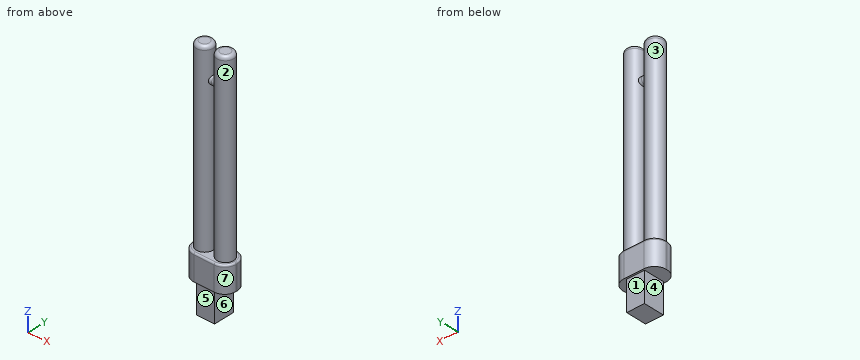
```python
from build123d import *

# Parameters (mm, degrees)
F0_R          = 6.096
F1_DEPTH      = 134.62
F2_R          = 2.921
F3_DEPTH      = 5.08
F3_DEPTH_BACK = 5.08
F4_R          = 2.54
F6_DEPTH      = 19.05
F7_R          = 1.27
F8_W          = 13.208
F8_H          = 15.24
F9_DEPTH      = 21.844


with BuildPart() as f1:
    # F0 (on Top) → F1 (new body)
    with BuildSketch(Plane.XY):
        with Locations((7.62, 0)):
            Circle(F0_R)
        with Locations((-7.62, 0)):
            Circle(F0_R)
    extrude(amount=F1_DEPTH)

    # F2 (on Right) → F3 (join, two sides)
    with BuildSketch(Plane.YZ) as f3_sk:
        with Locations((0, 111.602642)):
            Circle(F2_R)
    extrude(amount=F3_DEPTH)
    extrude(f3_sk.sketch, amount=-F3_DEPTH_BACK)

    # F4
    f4_edges = [f1.edges().sort_by_distance(p)[0] for p in [
        (-13.716, 0, 134.62),
        (1.524, 0, 134.62),
    ]]
    fillet(f4_edges, radius=F4_R)

    # F5 (on Top) → F6 (join)
    with BuildSketch(Plane.XY):
        with BuildLine():
            ThreePointArc((-15.875, -0.508), (-13.419969, -6.434969), (-7.493, -8.89))
            Line((-7.493, -8.89), (7.493, -8.89))
            ThreePointArc((7.493, -8.89), (13.419969, -6.434969), (15.875, -0.508))
            Line((15.875, -0.508), (15.875, 0.508))
            ThreePointArc((15.875, 0.508), (13.419969, 6.434969), (7.493, 8.89))
            Line((7.493, 8.89), (-7.493, 8.89))
            ThreePointArc((-7.493, 8.89), (-13.419969, 6.434969), (-15.875, 0.508))
            Line((-15.875, 0.508), (-15.875, -0.508))
        make_face()
    extrude(amount=-F6_DEPTH)

    # F7
    f7_edges = [f1.edges().sort_by_distance(p)[0] for p in [
        (0, -8.89, 0),
    ]]
    fillet(f7_edges, radius=F7_R)

    # F8 (on face) → F9 (join)
    with BuildSketch(Plane(origin=(0, 0, -19.05), x_dir=(1, 0, 0), z_dir=(0, 0, -1))):
        Rectangle(F8_W, F8_H)
    extrude(amount=F9_DEPTH)


solid = f1.part
```
Source: CAD feature listing. Evaluate the final solid. Frame: model axes, mm. Face numbers are marked on the shaded views. A direction names the side the tool comes from. Coordinates: 2 decimals unless noted, no trailing zeros. Loops run counter-clockwise (first coordinate to the right, second up) from the corner with the lowest first, then second, coordinate; pieces in that order, holes last. Notation, with made-up numbers: M -5,78.25 L 41,78.25 A24 cw 41,98.25 Z; hole C -39,27.5 d4. An arc over 180 degrees is marked long. Put each result on its own line as item: value. Start each with the question number.
1) Cut plane B-B on z = -21.5. Return the cut outline in (x, y).
2) Cut plane A-A on z = 100. Return the cut outline in (x, y), then the cut area to 3 significant figures.
3) Pull-direction query (X, two-part tool) for the marked faces 1, 2, 3 and 4; classes: pulls with the +X half, pulls with the -X half, needs draft (parallel to the pull), parting line crosses it, or undercut.
4) Ray query, L1, parallel to Z at x = 8.5, y = 0.5; L2, parallel to X at y = -4, z = 79; L3, parallel to X at y = 3.75, z = 3.5. Return the intervals inside material, ascending. Write a range as from..to.
5) Contact query for flat-ended pins moving along their axis: pin 1 Ø8 at (x, y) = (0, -2.5) entering from +Z; pin 2 Ø7.5 at (y, z) = (0.5, -31) entering from +X; pin 3 Ø10.5 at (x, z) = (0, -25.5) entering from +Y. Output: stop coordinate, or through.
6) Reachability of the marked faces 5, 6 and 7 from +Z, -Z, +X, -X, +Y, -Y: full face, straight path, thin tool, end or side. Return the list, or none.
The answers:
1. outline: M -6.6,-7.62 L 6.6,-7.62 L 6.6,7.62 L -6.6,7.62 Z
2. outline: C -7.62,0 d12.19; C 7.62,0 d12.19
2. area: 233 mm²
3. face 1: needs draft
3. face 2: undercut
3. face 3: undercut
3. face 4: pulls with the -X half
4. L1: z = -19.05..134.62
4. L2: x = -12.22..-3.02, 3.02..12.22
4. L3: x = -12.43..-2.81, 2.81..12.43
5. pin 1: stops at z = 134.58
5. pin 2: stops at x = 6.6
5. pin 3: stops at y = 7.62
6. face 5: -Z, +X, -X, -Y
6. face 6: -Z, +X, +Y, -Y
6. face 7: +Z, -Z, +X, -Y
